from build123d import *

# Parameters (mm, degrees)
SKETCH1_R           = 2.5019
BOSS_EXTRUDE1_DEPTH = 7.0104
SKETCH2_R           = 1.7526
BOSS_EXTRUDE2_DEPTH = 2.9972
SKETCH3_R           = 0.99949
CUT_EXTRUDE1_DEPTH  = 11.0076
SKETCH4_R           = 1.9939
CUT_EXTRUDE2_DEPTH  = 6.985


with BuildPart() as part:
    # Sketch1 → Boss-Extrude1 (new body)
    with BuildSketch(Plane(origin=(0, 0, 0), x_dir=(1, 0, 0), z_dir=(0, 1, 0))):
        Circle(SKETCH1_R)
    extrude(amount=BOSS_EXTRUDE1_DEPTH)

    # Sketch2 → Boss-Extrude2 (add)
    with BuildSketch(Plane(origin=(0, 7.0104, 0), x_dir=(1, 0, 0), z_dir=(0, 1, 0))):
        Circle(SKETCH2_R)
    extrude(amount=BOSS_EXTRUDE2_DEPTH)

    # Sketch3 → Cut-Extrude1 (cut, through all)
    with BuildSketch(Plane(origin=(0, 10.0076, 0), x_dir=(1, 0, 0), z_dir=(0, 1, 0))):
        Circle(SKETCH3_R)
    extrude(amount=-CUT_EXTRUDE1_DEPTH, mode=Mode.SUBTRACT)

    # Sketch4 → Cut-Extrude2 (cut)
    with BuildSketch(Plane.XZ):
        Circle(SKETCH4_R)
    extrude(amount=-CUT_EXTRUDE2_DEPTH, mode=Mode.SUBTRACT)


solid = part.part
Check sheet for the modelled part. Datum: model origin and axes. Units: mm. A direction names the side the tool comes from. Round coordinates to 2 decimals unless told otherwise and drop trailing zeros. Write each loop counter-clockwise with the first axis right and the second up, starting at its lowest first coordinate (ties: lowest second). Pieces come first, ordered by that corner, then holes. Notation, with made-up numbers: (-27, 46.5) - (-9, 46.5) arc R22 ccw to (-9, 76.5) - close; hole circle Ø5 at (79, 27). An arc over 180 degrees is marked (long way). Return JSON: item names as keys, results as strings.
Q1. Cross-section at B-B (z = 0). Record the boundary of the cut face in (x, y) (1 decimal).
Returned:
{"outline": "(-2.5, 0) - (-2, 0) - (-2, 7) - (-1, 7) - (-1, 10) - (-1.8, 10) - (-1.8, 7) - (-2.5, 7) - close; (1, 7) - (2, 7) - (2, 0) - (2.5, 0) - (2.5, 7) - (1.8, 7) - (1.8, 10) - (1, 10) - close"}
Q2. Cross-section at D-D (x = 1.35). Record the boundary of the cut face in (y, z) (3 decimals).
Returned:
{"outline": "(0, -2.106) - (7.01, -2.106) - (7.01, -1.118) - (10.008, -1.118) - (10.008, 1.118) - (7.01, 1.118) - (7.01, 2.106) - (0, 2.106) - (0, 1.467) - (6.985, 1.467) - (6.985, -1.467) - (0, -1.467) - close"}
Q3. Access from +Z, -Z, +X, -X, +Y, -Y to the whole of each face (thin tool, end or side, straight path). Record for faces 5 (the flat face through (-2, 0, 1)), 6 (the cylindrical face through (1.67, 8.49, -0.53)), 7 (the cylindrical face through (1.9, 3.4, 0.6)).
Returned:
{"face 5": "+Z, -Z, +X, -X, -Y", "face 6": "+Y", "face 7": "-Y"}
Q4. Cross-section at C-C (y = 4). Record the boundary of the cut face in (x, z), then the cut area to 3 significant figures.
Returned:
{"outline": "circle Ø5 at (0, 0); hole circle Ø3.99 at (0, 0)", "area": "7.17 mm²"}
Q5. Cross-section at A-A (x = 0). Record the boundary of the cut face in (y, z) (1 decimal).
Returned:
{"outline": "(0, -2.5) - (7, -2.5) - (7, -1.8) - (10, -1.8) - (10, -1) - (7, -1) - (7, -2) - (0, -2) - close; (0, 2) - (7, 2) - (7, 1) - (10, 1) - (10, 1.8) - (7, 1.8) - (7, 2.5) - (0, 2.5) - close"}
Q6. Draft check along Z on faces 1 (the flat face through (1, 6.985, -1)), 2 (the cylindrical face through (-2, 3.5, 1.5)), 3 (the flat face through (-2, 7.01, 1)), 4 (the cylindrical face through (1, 9, 0)). Enter one of: released by +Z, released by -Z, zero draft, split by the parting line, or undercut.
Returned:
{"face 1": "undercut", "face 2": "split by the parting line", "face 3": "zero draft", "face 4": "undercut"}
Q7. Scan lines: L1, parallel to Z at x = 0, y = 8.95; L2, parallel to Z at x = 0, y = 5.5. Record each from-to range of solid material in increasing order. Write a range as from..to.
Returned:
{"L1": "z = -1.75..-1, 1..1.75", "L2": "z = -2.5..-1.99, 1.99..2.5"}
